```python
from build123d import *

# Parameters (mm, degrees)
F0_W     = 83.50922
F0_H     = 17.687716
F1_DEPTH = 3.81


with BuildPart() as f1:
    # F0 (on Front) → F1 (new body)
    with BuildSketch(Plane.XZ):
        with Locations((0, 8.843858)):
            Rectangle(F0_W, F0_H)
        Polygon((41.75461, 17.687716), (41.75461, 0), (68.384546, 8.843858), align=None)
        Polygon((-68.384535, 8.843858), (-41.75461, 0), (-41.75461, 17.687716), align=None)
    extrude(amount=F1_DEPTH)


solid = f1.part
```
Build history of the part. All positions in model axes, mm. Coordinates: 2 decimals unless noted, no trailing zeros. Write each loop counter-clockwise with the first axis right and the second up, starting at its lowest first coordinate (ties: lowest second). Pieces come first, ordered by that corner, then holes.
1. Drill centre lines: probe 1 along Z at (x, y) = (-53, -0.95); probe 2 along Z at (x, y) = (-50, -2.15). Where is each one in solid material? Low to high.
Answer block:
probe 1: z = 3.73 to 13.95
probe 2: z = 2.74 to 14.95
2. Band-saw the part on C-C, the plane z = 6.75. Give the cut face in (x, y).
Answer block:
outline: (-62.08, -3.81) - (62.08, -3.81) - (62.08, 0) - (-62.08, 0) - close
3. Band-saw the part on B-B, the plane x = 57. Give the cut face in (y, z), and give its area (3 significant figures).
Answer block:
outline: (-3.81, 5.06) - (0, 5.06) - (0, 12.62) - (-3.81, 12.62) - close
area: 28.8 mm2
4. Band-saw the part on A-A, the plane y = -1.7. Give the cut face in (x, z).
Answer block:
outline: (-68.38, 8.84) - (-41.75, 0) - (41.75, 0) - (68.38, 8.84) - (41.75, 17.69) - (-41.75, 17.69) - close
